Here's how the part is built. I have some questions about the finished solid (model axes, mm). Round coordinates to 2 decimals unless told otherwise and drop trailing zeros. Order: outer loops, then holes, each group sorted by start corner. A loop starts at its lowest first (then second) coordinate and runs counter-clockwise, first axis right, second up. Notation, with made-up numbers: (-34, 14.5) -> (-8, 14.5) arc R4 cw to (-8, 18.5) -> close; hole circle Ø9 at (-10.75, 81). An arc over 180 degrees is marked (long way). Use a Markdown table: item, result. Add a question column.
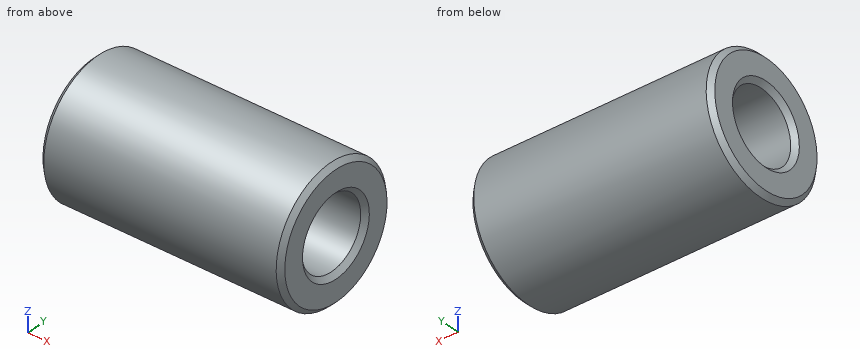
from build123d import *

# Parameters (mm, degrees)
SKETCH1_R           = 14
SKETCH1_R_2         = 7.5
BOSS_EXTRUDE1_DEPTH = 25.75
CHAMFER1_SIZE       = 1


with BuildPart() as part:
    # Sketch1 → Boss-Extrude1 (new, symmetric)
    with BuildSketch(Plane(origin=(0, 0, 0), x_dir=(0, -1, 0), z_dir=(1, 0, 0))):
        with Locations(Location((0, 0, 0), (0, 0, 90))):
            Circle(SKETCH1_R)
        with Locations(Location((0, 0, 0), (0, 0, 90))):
            Circle(SKETCH1_R_2, mode=Mode.SUBTRACT)
    extrude(amount=BOSS_EXTRUDE1_DEPTH, both=True)

    # Chamfer1
    chamfer1_edges = [part.edges().sort_by_distance(p)[0] for p in [
        (-25.75, 0, 14),
        (25.75, 0, 14),
        (-25.75, 0, 7.5),
        (25.75, 0, 7.5),
    ]]
    chamfer(chamfer1_edges, length=CHAMFER1_SIZE)


solid = part.part
(1) I want a section at C-C on x = -11. List the corners of the cut face in (y, z) for me, and give its area (3 significant figures).
(2) I'm going to push flat-ended pins straight in: P1, Ø5, axis at x = 5.5, y = -9.5, coming from the +Z side; P2, Ø1.5, axis at x = -0.5, z = 10, coming from the -Y side; P3, Ø13.5, axis at y = 0, z = 0, coming from the -X side; P4, Ø3, axis at x = 0, y = 3, coming from the +Z side. Where does each tip first touch, or does it pass through?
(3) I want a section at A-A on y = 0. List the corners of the cut face in (x, z) for me, and give its area (4 significant figures).
(4) Please list where these lines run through material, in increasing order: probe 1 along Y at (x, z) = (-2, 0); probe 2 along Y at (x, z) = (-19, 2.5). Write a range as from..to.
Output:
| question | item | result |
|---|---|---|
| 1 | outline | circle Ø28 at (0, 0); hole circle Ø15 at (0, 0) |
| 1 | area | 439 mm² |
| 2 | P1 | z = 12.12 |
| 2 | P2 | y = -10.51 |
| 2 | P3 | through |
| 2 | P4 | z = 13.92 |
| 3 | outline | (-25.75, -13) -> (-24.75, -14) -> (24.75, -14) -> (25.75, -13) -> (25.75, -8.5) -> (24.75, -7.5) -> (-24.75, -7.5) -> (-25.75, -8.5) -> close; (-25.75, 8.5) -> (-24.75, 7.5) -> (24.75, 7.5) -> (25.75, 8.5) -> (25.75, 13) -> (24.75, 14) -> (-24.75, 14) -> (-25.75, 13) -> close |
| 3 | area | 665.5 mm² |
| 4 | probe 1 | -14..-7.5, 7.5..14 |
| 4 | probe 2 | -13.77..-7.07, 7.07..13.77 |
